```python
from build123d import *

# Parameters (mm, degrees)
STOCK_DRIVEBLOCK_CNC_10MM_MASTER_1_OUTLI_R = 1.6
STOCK_DRIVEBLOCK_CNC_10MM_MASTER_1_DEPTH   = 2
STOCK_DRIVEBLOCK_CNC_10MM_MASTER_1_START   = 2
STOCK_DRIVEBLOCK_CNC_10MM_MASTER_1_2_OUT_R = 1.4
STOCK_DRIVEBLOCK_CNC_10MM_MASTER_1_2_DEPTH = 3
SKETCH1_W                                  = 34.3
SKETCH1_H                                  = 2
BOSS_EXTRUDE1_DEPTH                        = 3
BOSS_EXTRUDE2_DEPTH                        = 2
SKETCH3_W                                  = 8
SKETCH3_H                                  = 3
CUT_EXTRUDE1_DEPTH                         = 10


# Read off the part's stored shape, not the designer's step: Stock-driveblock-cnc-10mm-master-1
with BuildPart() as part:
    # Stock-driveblock-cnc-10mm-master-1 outli → Stock-driveblock-cnc-10mm-master-1 (new body)
    with BuildSketch(Plane.XY):
        with BuildLine():
            Line((21.15, -8.85), (21.15, 17.15))
            Line((21.15, 17.15), (17.15, 21.15))
            Line((17.15, 21.15), (-17.15, 21.15))
            Line((-17.15, 21.15), (-21.15, 17.15))
            Line((-21.15, 17.15), (-21.15, -8.85))
            ThreePointArc((-21.15, -8.85), (-20.564213562, -10.264213562), (-19.15, -10.85))
            Line((-19.15, -10.85), (-5.012733785, -10.85))
            ThreePointArc((-5.012733785, -10.85), (-4.525394068, -10.461803399), (-4.794788838, -9.9))
            ThreePointArc((-4.794788838, -9.9), (0, 11), (4.794788838, -9.9))
            ThreePointArc((4.794788838, -9.9), (4.525394068, -10.461803399), (5.012733785, -10.85))
            Line((5.012733785, -10.85), (19.15, -10.85))
            ThreePointArc((19.15, -10.85), (20.564213562, -10.264213562), (21.15, -8.85))
        make_face()
        with Locations((-15.5, 15.5)):
            Circle(STOCK_DRIVEBLOCK_CNC_10MM_MASTER_1_OUTLI_R, mode=Mode.SUBTRACT)
        with Locations((15.5, 15.5)):
            Circle(STOCK_DRIVEBLOCK_CNC_10MM_MASTER_1_OUTLI_R, mode=Mode.SUBTRACT)
    extrude(amount=STOCK_DRIVEBLOCK_CNC_10MM_MASTER_1_DEPTH)

    # Stock-driveblock-cnc-10mm-master-1 2 out → Stock-driveblock-cnc-10mm-master-1 2 (add)
    with BuildSketch(Plane.XY.offset(STOCK_DRIVEBLOCK_CNC_10MM_MASTER_1_START)):
        with Locations((-9.5, 8.75)):
            Circle(STOCK_DRIVEBLOCK_CNC_10MM_MASTER_1_2_OUT_R)
        with Locations((9.5, 8.75)):
            Circle(STOCK_DRIVEBLOCK_CNC_10MM_MASTER_1_2_OUT_R)
        with Locations((9.5, -8.75)):
            Circle(STOCK_DRIVEBLOCK_CNC_10MM_MASTER_1_2_OUT_R)
        with Locations((-9.5, -8.75)):
            Circle(STOCK_DRIVEBLOCK_CNC_10MM_MASTER_1_2_OUT_R)
    extrude(amount=STOCK_DRIVEBLOCK_CNC_10MM_MASTER_1_2_DEPTH)

    # Sketch1 → Boss-Extrude1 (add)
    with BuildSketch(Plane(origin=(0, 21.15, 0), x_dir=(1, 0, 0), z_dir=(0, 1, 0))):
        with Locations((0, -1)):
            Rectangle(SKETCH1_W, SKETCH1_H)
    extrude(amount=BOSS_EXTRUDE1_DEPTH)

    # Sketch2 → Boss-Extrude2 (add)
    with BuildSketch(Plane(origin=(0, 24.15, 0), x_dir=(1, 0, 0), z_dir=(0, 1, 0))):
        Polygon((9.45, -1.5), (10.95, -1.5), (10.95, 0), (6.05, 0), (6.05, -1.5), (7.55, -1.5), (7.55, -2), (9.45, -2), align=None)
        Polygon((-9.45, -1.5), (-9.45, -2), (-7.55, -2), (-7.55, -1.5), (-6.05, -1.5), (-6.05, 0), (-10.95, 0), (-10.95, -1.5), align=None)
    extrude(amount=BOSS_EXTRUDE2_DEPTH)

    # Sketch3 → Cut-Extrude1 (cut)
    with BuildSketch(Plane.XY.offset(2)):
        with Locations((0, 22.65)):
            Rectangle(SKETCH3_W, SKETCH3_H)
    extrude(amount=-CUT_EXTRUDE1_DEPTH, mode=Mode.SUBTRACT)


solid = part.part
```
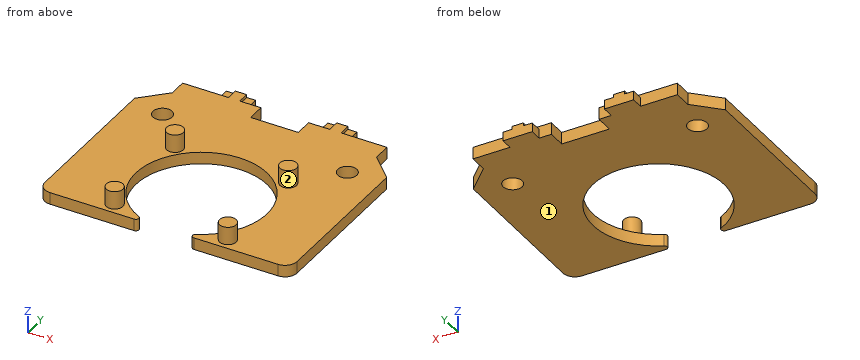
Geometry check sheet. Reference: the model listing, model coordinates, mm. Face numbers are marked on the shaded views. Coordinates: 2 decimals unless noted, no trailing zeros. Order: outer loops, then holes, each group sorted by start corner. A loop starts at its lowest first (then second) coordinate and runs counter-clockwise, first axis right, second up.
Q1. Draft check along X on the marked faces 1 and 2. Enter one of: released by +X, released by -X, zero draft, split by the parting line, or undercut.
Reply:
face 1: zero draft
face 2: undercut
Q2. Thickness scan on probe 1 along Y at (x, z) = (-15.5, 1.3); probe 2 along X at (y, z) = (0, 1.05); probe 3 along Y at (x, z) = (0, 0.85). Record the ranges inside material, lowest first.
Reply:
probe 1: y = -10.85 to 13.9, 17.1 to 24.15
probe 2: x = -21.15 to -11, 11 to 21.15
probe 3: y = 11 to 21.15
Q3. Sectioned sample at C-C on z = 3.35. Record the cut outline in (x, y).
Reply:
outline: circle Ø2.8 at (-9.5, -8.75); circle Ø2.8 at (-9.5, 8.75); circle Ø2.8 at (9.5, -8.75); circle Ø2.8 at (9.5, 8.75)
Q4. Sectioned sample at A-A on y = 22. Record the cut outline in (x, z), and give its area (3 significant figures).
Reply:
outline: (-17.15, 0) - (-4, 0) - (-4, 2) - (-17.15, 2) - close; (4, 0) - (17.15, 0) - (17.15, 2) - (4, 2) - close
area: 52.6 mm2
Q5. Sectioned sample at D-D on y = 15.5. Record the cut outline in (x, z).
Reply:
outline: (-21.15, 0) - (-17.1, 0) - (-17.1, 2) - (-21.15, 2) - close; (-13.9, 0) - (13.9, 0) - (13.9, 2) - (-13.9, 2) - close; (17.1, 0) - (21.15, 0) - (21.15, 2) - (17.1, 2) - close
Q6. Sectioned sample at B-B on x = -15.5. Record the cut outline in (y, z), and give its area (3 significant figures).
Reply:
outline: (-10.85, 0) - (13.9, 0) - (13.9, 2) - (-10.85, 2) - close; (17.1, 0) - (24.15, 0) - (24.15, 2) - (17.1, 2) - close
area: 63.6 mm2
Q7. Depth check by flat-ended pin: pin 1 Ø1.6 at (x, z) = (1, 1) entering from +Y; pin 2 Ø0.6 at (x, z) = (-14, 1.5) entering from +Y; pin 3 Ø1.6 at (y, z) = (25, 0.5) entering from -X. Enter the tip coordinate at first touch or a pass-through.
Reply:
pin 1: stops at y = 21.15
pin 2: stops at y = 24.15
pin 3: stops at x = -10.95
